from build123d import *

# Parameters (mm, degrees)
BOSS_EXTRUDE1_DEPTH      = 37.465
BOSS_EXTRUDE1_DEPTH_BACK = 37.465
SKETCH3_W                = 64.262
SKETCH3_H                = 110.648250087
CUT_EXTRUDE1_DEPTH       = 55.118
CUT_EXTRUDE1_DEPTH_BACK  = 109.601
SKETCH4_R                = 6.35
CUT_EXTRUDE2_DEPTH       = 109.601


with BuildPart() as part:
    # Sketch1 → Revolve1 (revolve)
    with BuildSketch(Plane.XY):
        Polygon((0, 57.15), (20.955, 57.15), (20.955, 54.61), (17.272, 54.61), (17.272, 0), (0, 0), align=None)
    revolve(axis=Axis((0, 38.1873125, 0), (0, -1, 0)))

    # Sketch2 → Boss-Extrude1 (add, two sides)
    with BuildSketch(Plane.XY) as boss_extrude1_sk:
        with BuildLine():
            Line((-25.4, 0), (25.4, 0))
            Line((25.4, 0), (25.4, -10.957312238))
            ThreePointArc((25.4, -10.957312238), (25.517902954, -12.683821415), (25.869422667, -14.378273814))
            Line((25.869422667, -14.378273814), (43.980577333, -79.129038424))
            ThreePointArc((43.980577333, -79.129038424), (38.222573525, -93.476838151), (22.872930676, -91.632270653))
            Line((22.872930676, -91.632270653), (-21.577069324, -48.186556851))
            ThreePointArc((-21.577069324, -48.186556851), (-24.405314614, -44.031314693), (-25.4, -39.104286198))
            Line((-25.4, -39.104286198), (-25.4, 0))
        make_face()
    extrude(amount=BOSS_EXTRUDE1_DEPTH)
    extrude(boss_extrude1_sk.sketch, amount=-BOSS_EXTRUDE1_DEPTH_BACK)

    # Sketch3 → Cut-Extrude1 (cut, two sides)
    with BuildSketch(Plane.ZY.offset(25.4)) as cut_extrude1_sk:
        with Locations((0, -60.404125044)):
            Rectangle(SKETCH3_W, SKETCH3_H)
    extrude(amount=CUT_EXTRUDE1_DEPTH, mode=Mode.SUBTRACT)
    extrude(cut_extrude1_sk.sketch, amount=-CUT_EXTRUDE1_DEPTH_BACK, mode=Mode.SUBTRACT)

    # Sketch4 → Cut-Extrude2 (cut)
    with BuildSketch(Plane.XY.offset(37.465)):
        with Locations((31.75, -82.55)):
            Circle(SKETCH4_R)
    extrude(amount=-CUT_EXTRUDE2_DEPTH, mode=Mode.SUBTRACT)


solid = part.part
Could you check a few things on this model? Use its own coordinates, in mm. A direction names the side the tool comes from. Give positions to 0.01 mm unless a question says otherwise; leave off trailing zeros. Write each loop counter-clockwise with the first axis right and the second up, starting at its lowest first coordinate (ties: lowest second). Pieces come first, ordered by that corner, then holes. Notation, with made-up numbers: (15.5, -32.5) - (37.5, -32.5) arc R28 cw to (37.5, 2.5) - close; hole circle Ø4 at (77, 0). An arc over 180 degrees is marked (long way). Use CSV: the item, a comma, the result in double quotes. Start each with the question number.
Item 1: If I drill on line 1 along Y through (x, z) = (11.5, 16.5); line 2 along Z through (x, y) = (21, -13) (3 decimals); line 3 along Y through (x, z) = (1.5, -0.5), over which ranges is the centre line in solid material (lowest first)?
Item 2: I want a section at C-C, the plane y = -82.55. Please give me the cut outline in (x, z) (3 decimals).
Item 3: I want a section at A-A, the plane y = -8. Please give me the cut outline in (x, z) (3 decimals).
Item 4: I want a section at D-D, the plane z = 27. Please give me the cut outline in (x, y).
Item 5: For faces 1 (the face through (-25.4, -4, 3)), 2 (the face through (3, 54.61, 17.2)), which set-ups out of +Z, -Z, +X, -X, +Y, -Y let a thin tool reach every point of the face, with its end or its side?
Item 6: I'm going to push flat-ended pins straight in: pin 1 (1 mm diameter, centred on x = -4.5, y = 15.5, fed in from +Z); pin 2 (3 mm diameter, centred on x = 10.5, z = -19, fed in from -Y); pin 3 (5.5 mm diameter, centred on y = -6, z = 5, fed in from +X). Where does each tip first touch, or does it pass through?
Item 7: I want a section at B-B, the plane x = 34. Please give me the cut outline in (y, z) (3 decimals), then the cut area to 3 significant figures.
Item 8: If we mould it in two halves opening along Z, with no side actions, what happens to faces 3 (the face through (-2.728, 55.862, 20.777)), 4 (the face through (9, -41, -32.131)), 5 (the face through (10, -47, -37.465)), 6 (the face through (25.4, -3, 1))? For each: pulls with the +Z half, pulls with the -Z half, needs draft (parallel to the pull), parting line crosses it, or undercut.
Findings:
1,line 1,"y = -5.08 to 0, 54.61 to 57.15"
1,line 2,"z = -37.465 to -32.131, 32.131 to 37.465"
1,line 3,"y = -5.08 to 57.15"
2,outline,"(13.581, -37.465) - (25.4, -37.465) - (25.4, -32.131) - (13.581, -32.131) - close; (13.581, 32.131) - (25.4, 32.131) - (25.4, 37.465) - (13.581, 37.465) - close; (38.1, -37.465) - (44.45, -37.465) - (44.45, -32.131) - (38.1, -32.131) - close; (38.1, 32.131) - (44.45, 32.131) - (44.45, 37.465) - (38.1, 37.465) - close"
3,outline,"(-25.4, -37.465) - (25.4, -37.465) - (25.4, -32.131) - (-25.4, -32.131) - close; (-25.4, 32.131) - (25.4, 32.131) - (25.4, 37.465) - (-25.4, 37.465) - close"
4,outline,"(-25.4, -5.08) - (25.4, -5.08) - (25.4, 0) - (-25.4, 0) - close"
5,face 1,"+Z, -Z, -X, +Y, -Y"
5,face 2,"none"
6,pin 1,"stops at z = 16.8"
6,pin 2,"stops at y = -5.08"
6,pin 3,"stops at x = 25.4"
7,outline,"(-95.049, -37.465) - (-88.488, -37.465) - (-88.488, -32.131) - (-95.049, -32.131) - close; (-95.049, 32.131) - (-88.488, 32.131) - (-88.488, 37.465) - (-95.049, 37.465) - close; (-76.612, -37.465) - (-43.447, -37.465) - (-43.447, -32.131) - (-76.612, -32.131) - close; (-76.612, 32.131) - (-43.447, 32.131) - (-43.447, 37.465) - (-76.612, 37.465) - close"
7,area,"424 mm2"
8,face 3,"parting line crosses it"
8,face 4,"undercut"
8,face 5,"pulls with the -Z half"
8,face 6,"needs draft"
